Could you check a few things on this model? Use its own coordinates, in mm. A direction names the side the tool comes from. Give positions to 0.01 mm unless a question says otherwise; leave off trailing zeros. Loops run counter-clockwise (first coordinate to the right, second up) from the corner with the lowest first, then second, coordinate; pieces in that order, holes last. Notation, with made-up numbers: (85.25, 12) -> (104.25, 12) arc R14 ccw to (104.25, 26) -> close; hole circle Ø11 at (40.25, 79). An arc over 180 degrees is marked (long way). Put each result on its own line as item: value.
```python
from build123d import *

# Parameters (mm, degrees)
F0_W     = 52.3490961641
F0_H     = 100.1019440591
F1_DEPTH = 15
F2_W     = 26.3490961641
F2_H     = 12
F3_DEPTH = 20
F5_DEPTH = 12
F7_DEPTH = 26.3
F10_D    = 12
F12_D    = 20


with BuildPart() as f1:
    # F0 (on Top) → F1 (new body)
    with BuildSketch(Plane.XY):
        with BuildLine():
            Line((26.4400355518, 50.134152174), (26.4692548662, 50.134152174))
            ThreePointArc((26.4692548662, 50.134152174), (0.280097127, 76.1836339389), (-25.9090606123, 50.134152174))
            Line((-25.9090606123, 50.134152174), (26.4400355518, 50.134152174))
        make_face()
        with Locations((0.2654874697, 0.0831801444)):
            Rectangle(F0_W, F0_H)
        with BuildLine():
            Line((26.4400355518, -49.9677918851), (-25.9090606123, -49.9677918851))
            ThreePointArc((-25.9090606123, -49.9677918851), (0.2654874697, -76.1423399672), (26.4400355518, -49.9677918851))
        make_face()
    extrude(amount=-F1_DEPTH)

    # F2 (on Top) → F3 (join)
    with BuildSketch(Plane.XY):
        with Locations((0.2654874697, -29.4927601161)):
            Rectangle(F2_W, F2_H)
    extrude(amount=F3_DEPTH)

    # F4 (on face) → F5 (join)
    with BuildSketch(Plane.XZ.offset(35.4927601161)):
        with BuildLine():
            Line((-12.9090606123, 20), (13.4400355518, 20))
            ThreePointArc((13.4400355518, 20), (0.2654874697, 33.1745480821), (-12.9090606123, 20))
        make_face()
    extrude(amount=-F5_DEPTH)

    # F6 (on face) → F7 (join)
    with BuildSketch(Plane.YZ.offset(13.4400355518)):
        with BuildLine():
            add(Edge.make_bspline(
                [(-23.4927601161, 12.5284092501), (-21.2797119115, 8.3236057962), (-15.6986097687, 3.625344109), (-5.9415775516, 4.0916807862), (0, 4.2679198086)],
                knots=[0, 0, 0, 0, 0.4600140191, 1, 1, 1, 1], degree=3))
            Line((-23.4927601161, 12.5284092501), (-23.4927601161, 0))
            Line((-23.4927601161, 0), (0, 0))
            Line((0, 0), (0, 4.2679198086))
        make_face()
    extrude(amount=-F7_DEPTH)

    # F8: F1 across plane


with BuildPart() as f1_1:
    add(f1.part)
    add(f1.part.mirror(Plane.XZ))

    # F10 (through all)
    with Locations(Plane.XZ.offset(35.4927601161)):
        with Locations((0, 20)):
            Hole(F10_D / 2)

    # F12 (through all)
    with Locations(Plane.XY):
        with Locations((0, 50.134152174), (0, -50.134152174)):
            Hole(F12_D / 2)


solid = f1_1.part
```
1. If we section it at D-D (x = 17): List the corners of the cut face in (y, z) for me.
Recorded:
outline: (-70.15, -15) -> (70.15, -15) -> (70.15, 0) -> (-70.15, 0) -> close
2. Thinking about a two-plate mould opening in X: for faces 1 (the face through (13.44, 0, 3)), 2 (the face through (2.168, 40.372, -7.605)), 3 (the face through (-12.909, -30, 10)), 4 (the face through (0, 23.493, 28)), which applies, pulls with the +X half, pulls with the -X half, needs draft (parallel to the pull), parting line crosses it, or undercut?
Recorded:
face 1: pulls with the +X half
face 2: undercut
face 3: pulls with the -X half
face 4: needs draft
3. I need wall thicknesses on line 1 (Y direction, x = 0, z = -8.75); line 2 (Z direction, x = 0, y = 28.25); line 3 (Z direction, x = 12, y = -24). Which ranges of each line are inside material? Lowest first, please.
Recorded:
line 1: y = -76.18 to -60.13, -40.13 to 40.13, 60.13 to 76.18
line 2: z = -15 to 14, 26 to 33.17
line 3: z = -15 to 25.99
4. For faces 5 (the face through (0, 35.493, 13)), 6 (the face through (0, -35.493, 13)), 7 (the face through (-12.909, 30, 10)), which set-ups out of +Z, -Z, +X, -X, +Y, -Y let a thin tool reach every point of the face, with its end or its side?
Recorded:
face 5: +Z, +X, -X, +Y
face 6: +Z, +X, -X, -Y
face 7: +Z, -X, +Y, -Y
5. If we section it at B-B (z = -4.5): Count the separate pieces of the cut face and the enclosed holes in it, then the cut area to 3 significant figures.
Recorded:
separate pieces: 1
enclosed holes: 2
area: 6,760 mm^2
6. I'm going to push flat-ended pins straight in: pin 1 (6.5 mm diameter, centred on y = 8.5, z = 6.5, fed in from -X); pin 2 (21 mm diameter, centred on x = 4.5, z = 25, fed in from +Y); pin 3 (8 mm diameter, centred on x = -5, z = 16, fed in from -Y). Where does each tip first touch, or does it pass through?
Recorded:
pin 1: stops at x = -12.86
pin 2: stops at y = 35.49
pin 3: stops at y = -35.49
7. If we section it at C-C (y = 46): List the corners of the cut face in (x, z) for me.
Recorded:
outline: (-25.91, -15) -> (-9.11, -15) -> (-9.11, 0) -> (-25.91, 0) -> close; (9.11, -15) -> (26.44, -15) -> (26.44, 0) -> (9.11, 0) -> close
8. If we section it at A-A (z = 24): List the corners of the cut face in (x, y) for me, then the cut area to 3 significant figures.
Recorded:
outline: (-12.29, -35.49) -> (-4.47, -35.49) -> (-4.47, -23.49) -> (-12.29, -23.49) -> close; (-12.29, 23.49) -> (-4.47, 23.49) -> (-4.47, 35.49) -> (-12.29, 35.49) -> close; (4.47, -35.49) -> (12.82, -35.49) -> (12.82, -23.49) -> (4.47, -23.49) -> close; (4.47, 23.49) -> (12.82, 23.49) -> (12.82, 35.49) -> (4.47, 35.49) -> close
area: 388 mm^2
